from build123d import *

# Parameters (mm, degrees)
SKETCH1_W           = 62
SKETCH1_H           = 65
BOSS_EXTRUDE1_DEPTH = 10
SKETCH2_W           = 12
SKETCH2_H           = 35
SKETCH2_W_2         = 11
SKETCH2_H_2         = 12
CUT_EXTRUDE2_DEPTH  = 47.013584951


with BuildPart() as part:
    # Sketch1 → Boss-Extrude1 (new body)
    with BuildSketch(Plane(origin=(0, 0, 0), x_dir=(0, 0, -1), z_dir=(1, 0, 0))):
        Rectangle(SKETCH1_W, SKETCH1_H)
    extrude(amount=BOSS_EXTRUDE1_DEPTH)

    # Sketch2 → Cut-Extrude2 (cut, through all)
    with BuildSketch(Plane(origin=(10, 0, 0), x_dir=(0, 0, -1), z_dir=(1, 0, 0))):
        with Locations((-25, -15)):
            Rectangle(SKETCH2_W, SKETCH2_H)
        Polygon((18.6, -20.5), (21, -20.5), (21, -32.5), (11, -32.5), (11, -20.5), (13.4, -20.5), (13.4, -15.5), (12, -15.5), (12, -9.5), (13.4, -9.5), (13.4, -0.5), (18.6, -0.5), (18.6, -9.5), (20, -9.5), (20, -15.5), (18.6, -15.5), align=None)
        Polygon((-19, 12.5), (-31, 12.5), (-31, 22.5), (-19, 22.5), (-19, 20.1), (-14, 20.1), (-14, 21.5), (-8, 21.5), (-8, 20.1), (1, 20.1), (1, 14.9), (-8, 14.9), (-8, 13.5), (-14, 13.5), (-14, 14.9), (-19, 14.9), align=None)
        with Locations((-4.5, -26.5)):
            Rectangle(SKETCH2_W_2, SKETCH2_H_2)
    extrude(amount=-CUT_EXTRUDE2_DEPTH, mode=Mode.SUBTRACT)


solid = part.part
Here's how the part is built. I have some questions about the finished solid (model axes, mm). A direction names the side the tool comes from. Round coordinates to 2 decimals unless told otherwise and drop trailing zeros. Loops run counter-clockwise (first coordinate to the right, second up) from the corner with the lowest first, then second, coordinate; pieces in that order, holes last. Notation, with made-up numbers: (44.25, 34) - (90.25, 34) arc R20 cw to (90.25, 40) - close; hole circle Ø4 at (28, 68). An arc over 180 degrees is marked (long way). One line per question, with ' | ' between items. Start each with the question number.
Q1. I want a section at A-A (z = 15.5). Write out the boundary of the cut face in (x, y).
Q2. Will these pins go through, and if not, where does the flat tip stop? pin 1 (1.5 mm diameter, centred on x = 7, y = -21, fed in from +Z); pin 2 (10 mm diameter, centred on y = -15, z = 10.5, fed in from -X); pin 3 (1.6 mm diameter, centred on x = 4, z = -15.5, fed in from -Y); pin 4 (2.5 mm diameter, centred on x = 4, z = 4.5, fed in from -Y).
Q3. I want a section at B-B (y = -4). Write out the boundary of the cut face in (x, z).
Q4. We'd pull the mould along Y, two halves only. Please class faces 1 (the flat face through (5, -18, -18.6)), 2 (the flat face through (5, -20.5, -12)), 3 (the flat face through (5, -15.5, -13)): +Y half, -Y half, draft (parallel to the pull), parting line (faces both ways), or undercut.
Q5. Please list where these lines run through material, in increasing order: line 1 (Z direction, x = 6.5, y = -26.5); line 2 (Z direction, x = 7.5, y = -11); line 3 (Y direction, x = 7.75, z = 1.5). Write a range as [from, to].
Q6. I want a section at C-C (z = -16). Write out the boundary of the cut face in (x, y), then the cut area to 3 significant figures.
Q7. For faces 4 (the flat face through (5, 13.5, 11)), 5 (the flat face through (5, -0.5, -16)), 6 (the flat face through (5, 14, 19)), which set-ups out of +Z, -Z, +X, -X, +Y, -Y let a thin tool reach every point of the face, with its end or its side?
Response values:
1) outline: (0, -32.5) - (10, -32.5) - (10, 14.9) - (0, 14.9) - close; (0, 20.1) - (10, 20.1) - (10, 32.5) - (0, 32.5) - close
2) pin 1: stops at z = 19 | pin 2: stops at x = 0 | pin 3: stops at y = -0.5 | pin 4: stops at y = -20.5
3) outline: (0, -31) - (10, -31) - (10, -18.6) - (0, -18.6) - close; (0, -13.4) - (10, -13.4) - (10, 19) - (0, 19) - close
4) face 1: draft | face 2: -Y half | face 3: undercut
5) line 1: z = [-31, -21], [-11, -1], [10, 19] | line 2: z = [-31, -20], [-12, 19] | line 3: y = [-20.5, 14.9], [20.1, 32.5]
6) outline: (0, -0.5) - (10, -0.5) - (10, 32.5) - (0, 32.5) - close | area: 330 mm²
7) face 4: +X, -X | face 5: +X, -X, -Y | face 6: +Z, +X, -X
